Part model, mm, in its own coordinate system. Face numbers are marked on the shaded views. A direction names the side the tool comes from. Round coordinates to 2 decimals unless told otherwise and drop trailing zeros. Loops run counter-clockwise (first coordinate to the right, second up) from the corner with the lowest first, then second, coordinate; pieces in that order, holes last.
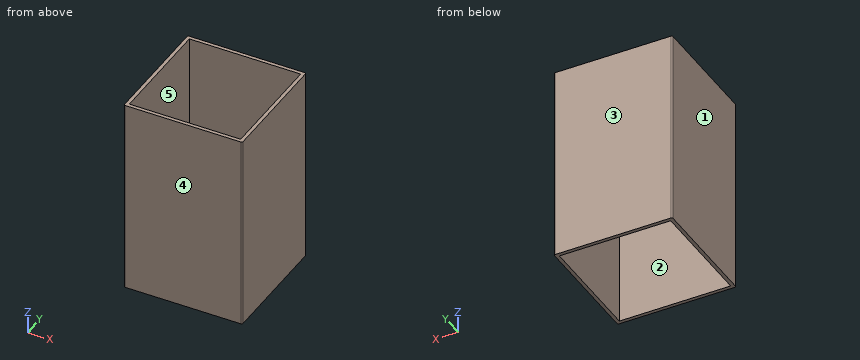
from build123d import *

# Parameters (mm, degrees)
F0_W     = 30
F0_H     = 50
F1_DEPTH = 30
F2_W     = 28.2
F2_H     = 28.2
F3_DEPTH = 50.001
F4_R     = 0.3


with BuildPart() as f1:
    # F0 (on Front) → F1 (new body)
    with BuildSketch(Plane.XZ):
        with Locations((0.765305, 25)):
            Rectangle(F0_W, F0_H)
    extrude(amount=F1_DEPTH)

    # F2 (on face) → F3 (cut, through all)
    with BuildSketch(Plane.XY.offset(50)):
        with Locations((0.765305, -15)):
            Rectangle(F2_W, F2_H)
    extrude(amount=-F3_DEPTH, mode=Mode.SUBTRACT)

    # F4
    f4_edges = [f1.edges().sort_by_distance(p)[0] for p in [
        (15.765305, -30, 25),
        (15.765305, 0, 25),
        (-14.234695, 0, 25),
        (-14.234695, -30, 25),
    ]]
    fillet(f4_edges, radius=F4_R)


solid = f1.part
1) Slice it at B-B, the plane y = -19. Give the cut face in (x, z), then the cut area to 3 significant figures.
Values:
outline: (-14.23, 0) - (-13.33, 0) - (-13.33, 50) - (-14.23, 50) - close; (14.87, 0) - (15.77, 0) - (15.77, 50) - (14.87, 50) - close
area: 90.0 mm2
2) Mould opens along X. For the marked faces 1, 2 and 3 say: released by +X, released by -X, zero draft, split by the parting line, or undercut.
Values:
face 1: released by -X
face 2: undercut
face 3: zero draft
3) Tool access for the marked faces 4 and 5: list every direction of +Z, -Z, +X, -X, +Y, -Y with a clear straight run to the whole face (end or side of a thin tool).
Values:
face 4: +Z, -Z, +X, -X, -Y
face 5: +Z, -Z
4) Drop a flat-ended pin along its axis: pin 1 Ø8 at (x, y) = (-10, -17.5) entering from +Z. Give the stop position or say it passes through.
Values:
pin 1: stops at z = 50
5) Slice it at C-C, the plane z = 31. Give the cut face in (x, y).
Values:
outline: (-14.23, -29.7) arc R0.3 ccw to (-13.93, -30) - (15.47, -30) arc R0.3 ccw to (15.77, -29.7) - (15.77, -0.3) arc R0.3 ccw to (15.47, 0) - (-13.93, 0) arc R0.3 ccw to (-14.23, -0.3) - close; hole (-13.33, -29.1) - (14.87, -29.1) - (14.87, -0.9) - (-13.33, -0.9) - close
6) Slice it at A-A, the plane x = -4.75. Give the cut face in (y, z).
Values:
outline: (-30, 0) - (-29.1, 0) - (-29.1, 50) - (-30, 50) - close; (-0.9, 0) - (0, 0) - (0, 50) - (-0.9, 50) - close
7) Wall check: line 1 along Y through (x, z) = (-10.25, 21); line 2 along X through (y, z) = (-19, 38). Give the ranges that are in metal, low to high.
Values:
line 1: y = -30 to -29.1, -0.9 to 0
line 2: x = -14.23 to -13.33, 14.87 to 15.77
